from build123d import *

# Parameters (mm, degrees)
F1_DEPTH = 3
F2_D     = 3


# Not quite as in the source:
# - a feature of the source that left no trace in its solid (it failed there, or was rolled back) is left out


with BuildPart() as f1:
    # F0 (on Front) → F1 (new body)
    with BuildSketch(Plane.XZ):
        with BuildLine():
            ThreePointArc((6.3713843202, -7.1733870463), (5.0414339245, -1.2687792727), (5.5912292227, 4.7587315024))
            Line((5.5912292227, 4.7587315024), (12.9146554895, 33.77647678))
            ThreePointArc((12.9146554895, 33.77647678), (9.290190371, 39.8479883385), (3.2186788125, 36.22352322))
            Line((3.2186788125, 36.22352322), (-4.1047474542, 7.2057779424))
            ThreePointArc((-4.1047474542, 7.2057779424), (-4.9372598224, -1.9212140236), (-2.9234191128, -10.8621035089))
            Line((-2.9234191128, -10.8621035089), (3.4192654345, -26.8443582313))
            ThreePointArc((3.4192654345, -26.8443582313), (9.9110253823, -29.6474017165), (12.7140688675, -23.1556417687))
            Line((12.7140688675, -23.1556417687), (6.3713843202, -7.1733870463))
        make_face()
    extrude(amount=F1_DEPTH)

    # F2 (through all)
    with Locations(Plane(origin=(0, 0, 0), x_dir=(1, 0, 0), z_dir=(0, 1, 0))):
        with Locations((8.066667151, -35), (8.066667151, 25)):
            Hole(F2_D / 2)


solid = f1.part
Build history of the part. All positions in model axes, mm. A direction names the side the tool comes from. Round coordinates to 2 decimals unless told otherwise and drop trailing zeros. Loops run counter-clockwise (first coordinate to the right, second up) from the corner with the lowest first, then second, coordinate; pieces in that order, holes last. Notation, with made-up numbers: (70, 88) -> (112, 88) arc R20 cw to (112, 123) -> close; hole circle Ø3 at (-4, 21). An arc over 180 degrees is marked (long way). One line per item, written item: value. Start each with the question number.
Q1. Cut at C-C on z = 35. List the corners of the cut face in (x, y), plus the area to 3 significant figures.
Q2. Two-plate mould, pull along X, no slides. Class faces 3 (the face through (9.2, -1.48, 19.06)), 4 (the face through (-0.39, -1.48, 21.92)), 5 (the face through (8.262, -1.521, -26.487)): released by +X, released by -X, zero draft, split by the parting line, or undercut.
Q3. Cut at A-A on z = -25. List the corners of the cut face in (x, y).
Q4. 3-axis set-ups, long thin cutter, end or side, ignore diameter. For faces 1 (the face through (9.59, -1.48, -15.28)), 2 (the face through (-4.945, -1.479, -1.793)): which of +Z, -Z, +X, -X, +Y, -Y reach the whole face in a straight line?
Q5. Probe line 1 along X through (y, z) = (-0.8, -25); line 2 along X through (y, z) = (-1.55, 35); line 3 along X through (y, z) = (-0.7, 23.5). List the from-to ranges inside material, lowest first.
Q6. Cut at D-D on x = 2.25. List the corners of the cut face in (y, z).
Q7. Drop flat-ended pins along their axis: pin 1 Ø1 at (y, z) = (-0.5, -10) entering from -X; pin 2 Ø1.8 at (x, z) = (8.07, -25) entering from +Y. Give the stop position or say it passes through.
Computed:
1. outline: (2.91, -3) -> (6.57, -3) -> (6.57, 0) -> (2.91, 0) -> close; (9.57, -3) -> (13.07, -3) -> (13.07, 0) -> (9.57, 0) -> close
1. area: 21.5 mm²
2. face 3: released by +X
2. face 4: released by -X
2. face 5: undercut
3. outline: (2.69, -3) -> (6.57, -3) -> (6.57, 0) -> (2.69, 0) -> close; (9.57, -3) -> (13.07, -3) -> (13.07, 0) -> (9.57, 0) -> close
4. face 1: +X, +Y, -Y
4. face 2: -X, +Y, -Y
5. line 1: 2.69 to 6.57, 9.57 to 13.07
5. line 2: 2.91 to 6.57, 9.57 to 13.07
5. line 3: 0.01 to 10.32
6. outline: (-3, -23.9) -> (0, -23.9) -> (0, 32.39) -> (-3, 32.39) -> close
7. pin 1: x = -3.43
7. pin 2: through
